from build123d import *

# Parameters (mm, degrees)
BOSS_EXTRUDE1_DEPTH      = 25
CUT_EXTRUDE1_DEPTH       = 4
FILLET1_R                = 4
FILLET2_R                = 10
FILLET3_R                = 5
FILLET4_R                = 3
BOSS_EXTRUDE2_DEPTH      = 3
BOSS_EXTRUDE2_DEPTH_BACK = 3
FILLET5_R                = 3
SKETCH6_W                = 13
SKETCH6_H                = 14
BOSS_EXTRUDE3_DEPTH      = 20
BOSS_EXTRUDE4_DEPTH      = 20
SKETCH9_W                = 13
SKETCH9_H                = 2
BOSS_EXTRUDE5_DEPTH      = 8
SKETCH7_W                = 13
SKETCH7_H                = 2
CUT_EXTRUDE2_DEPTH       = 5
SKETCH11_R               = 1.6
CUT_EXTRUDE3_DEPTH       = 19
CUT_EXTRUDE4_START       = -2
SKETCH12_R               = 1.6
CUT_EXTRUDE4_DEPTH       = 2
CUT_EXTRUDE5_DEPTH       = 6.5
CUT_EXTRUDE5_DEPTH_BACK  = 6.5
CUT_EXTRUDE6_START       = -17
SKETCH15_R               = 6.5
CUT_EXTRUDE6_DEPTH       = 17


with BuildPart() as part:
    # Sketch1 → Boss-Extrude1 (new body)
    with BuildSketch(Plane(origin=(0, 0, 0), x_dir=(0, 0, -1), z_dir=(1, 0, 0))):
        Polygon((0, 0), (-130, 0), (-130, 5), (-100.000366453, 5.148280317), (-77.868517379, 27.5), (101.088229162, 27.5), (114, 18), (114, 0), (74, 0), (74, 7.5), (0, 7.5), align=None)
    extrude(amount=BOSS_EXTRUDE1_DEPTH)

    # Sketch4 → Cut-Extrude1 (cut)
    with BuildSketch(Plane(origin=(25, 0, 0), x_dir=(0, 0, -1), z_dir=(1, 0, 0))):
        Polygon((-100.876178749, 0), (0, 0), (111, 0), (111, 3), (111, 16.482758557), (100.103496394, 24.5), (-76.617181678, 24.5), align=None)
    cut_extrude1 = extrude(amount=-CUT_EXTRUDE1_DEPTH, mode=Mode.SUBTRACT)

    # Mirror2: Cut-Extrude1 across plane
    add(cut_extrude1.mirror(Plane(origin=(12.5, 0, 0), x_dir=(0, 0, 1), z_dir=(1, 0, 0))), mode=Mode.SUBTRACT)

    # Fillet1
    fillet1_edges = [part.edges().sort_by_distance(p)[0] for p in [
        (12.5, 7.5, -74),
        (12.5, 7.5, 0),
    ]]
    fillet(fillet1_edges, radius=FILLET1_R)

    # Fillet2
    fillet2_edges = [part.edges().sort_by_distance(p)[0] for p in [
        (23, 0, 100.876178749),
        (23, 24.5, 76.617181678),
        (23, 24.5, -100.103496394),
        (23, 16.482758557, -111),
        (2, 0, 100.876178749),
        (2, 16.482758557, -111),
        (2, 24.5, -100.103496394),
        (2, 24.5, 76.617181678),
    ]]
    fillet(fillet2_edges, radius=FILLET2_R)

    # Fillet3
    fillet3_edges = [part.edges().sort_by_distance(p)[0] for p in [
        (12.5, 5.148280317, 100.000366453),
        (12.5, 27.5, 77.868517379),
        (12.5, 27.5, -101.088229162),
        (12.5, 18, -114),
    ]]
    fillet(fillet3_edges, radius=FILLET3_R)

    # Fillet4
    fillet4_edges = [part.edges().sort_by_distance(p)[0] for p in [
        (0, 2.5, 130),
        (25, 2.5, 130),
    ]]
    fillet(fillet4_edges, radius=FILLET4_R)

    # Sketch5 → Boss-Extrude2 (add, two sides: drawn at the far end of the back side and taken through both)
    with BuildSketch(Plane(origin=(12.5, 0, 0), x_dir=(0, 0, -1), z_dir=(1, 0, 0)).offset(-BOSS_EXTRUDE2_DEPTH_BACK)):
        Polygon((-117.8659777, 5.059975288), (-103.793914836, 19.271838176), (-72.605250228, 19.271838176), (-95.8659777, 5.059975288), align=None)
    extrude(amount=BOSS_EXTRUDE2_DEPTH + BOSS_EXTRUDE2_DEPTH_BACK)

    # Fillet5
    fillet5_edges = [part.edges().sort_by_distance(p)[0] for p in [
        (12.5, 19.271838176, 103.793914836),
    ]]
    fillet(fillet5_edges, radius=FILLET5_R)

    # Sketch6 → Boss-Extrude3 (add)
    with BuildSketch(Plane.XZ):
        Polygon((0, -111), (4, -111), (4, -93), (21, -93), (21, -111), (25, -111), (25, -114), (0, -114), align=None)
        with Locations((12.5, -102)):
            Rectangle(SKETCH6_W, SKETCH6_H, mode=Mode.SUBTRACT)
    extrude(amount=BOSS_EXTRUDE3_DEPTH)

    # Sketch8 → Boss-Extrude4 (add)
    with BuildSketch(Plane.XZ):
        Polygon((21, 85), (4, 85), (4, 64), (6, 64), (6, 83), (19, 83), (19, 64), (21, 64), align=None)
    extrude(amount=BOSS_EXTRUDE4_DEPTH)

    # Sketch9 → Boss-Extrude5 (add)
    with BuildSketch(Plane.XZ):
        with Locations((12.5, 65)):
            Rectangle(SKETCH9_W, SKETCH9_H)
    extrude(amount=BOSS_EXTRUDE5_DEPTH)

    # Sketch7 → Cut-Extrude2 (cut)
    with BuildSketch(Plane.XZ.offset(20)):
        with Locations((12.5, -94)):
            Rectangle(SKETCH7_W, SKETCH7_H)
    extrude(amount=-CUT_EXTRUDE2_DEPTH, mode=Mode.SUBTRACT)

    # Sketch11 → Cut-Extrude3 (cut)
    with BuildSketch(Plane(origin=(0, 0, -114), x_dir=(-1, 0, 0), z_dir=(0, 0, -1))):
        with Locations((-15.75, -16.25)):
            Circle(SKETCH11_R)
        with Locations((-15.75, -8.75)):
            Circle(SKETCH11_R)
        with Locations((-9.25, -8.75)):
            Circle(SKETCH11_R)
        with Locations((-9.25, -16.25)):
            Circle(SKETCH11_R)
    extrude(amount=-CUT_EXTRUDE3_DEPTH, mode=Mode.SUBTRACT)

    # Sketch12 → Cut-Extrude4 (cut)
    with BuildSketch(Plane.XY.offset(85).offset(CUT_EXTRUDE4_START)):
        with Locations(Location((15.75, -16.25, 0), (0, 0, 180))):
            Circle(SKETCH12_R)
        with Locations(Location((9.25, -16.25, 0), (0, 0, 180))):
            Circle(SKETCH12_R)
        with Locations(Location((9.25, -8.75, 0), (0, 0, 180))):
            Circle(SKETCH12_R)
        with Locations(Location((15.75, -8.75, 0), (0, 0, 180))):
            Circle(SKETCH12_R)
    extrude(amount=CUT_EXTRUDE4_DEPTH, mode=Mode.SUBTRACT)

    # Sketch14 → Cut-Extrude5 (cut, two sides: drawn at the far end of the back side and taken through both)
    with BuildSketch(Plane(origin=(12.5, 0, 0), x_dir=(0, 0, -1), z_dir=(1, 0, 0)).offset(-CUT_EXTRUDE5_DEPTH_BACK)):
        Polygon((-83, 0), (-83, 13.475167258), (-72.975167258, 23.5), (95.592427597, 23.5), (109, 10.092427597), (109, 0), (95, 0), (95, 3.57939317), (87.07939317, 11.5), (-5.825100808, 11.5), (-13.325100808, 4), (-66, 4), (-66, 0), align=None)
    extrude(amount=CUT_EXTRUDE5_DEPTH + CUT_EXTRUDE5_DEPTH_BACK, mode=Mode.SUBTRACT)

    # Sketch15 → Cut-Extrude6 (cut)
    with BuildSketch(Plane.ZY.offset(-4).offset(CUT_EXTRUDE6_START)):
        with Locations((-91, 16)):
            Circle(SKETCH15_R)
        with Locations((-39.333333333, 16)):
            Circle(SKETCH15_R)
        with Locations((64, 16)):
            Circle(SKETCH15_R)
        with Locations((12.333333333, 16)):
            Circle(SKETCH15_R)
    extrude(amount=CUT_EXTRUDE6_DEPTH, mode=Mode.SUBTRACT)


solid = part.part
Build history of the part. All positions in model axes, mm. A direction names the side the tool comes from. Give positions to 0.01 mm unless a question says otherwise; leave off trailing zeros. Order: outer loops, then holes, each group sorted by start corner. A loop starts at its lowest first (then second) coordinate and runs counter-clockwise, first axis right, second up. Notation, with made-up numbers: M 78.25,77.25 L 116.25,77.25 A10 ccw 116.25,95.25 Z; hole C 60.25,84.25 d11. An arc over 180 degrees is marked long. Use one line per item in the form item = value.
1) Probe probe 1 along Z at (x, y) = (13.5, -6); probe 2 along X at (y, z) = (4, 77); probe 3 along Y at (x, z) = (17.5, 34). List the from-to ranges inside material, lowest first.
Calculated:
probe_1 = -114 to -109, -95 to -93, 64 to 66, 83 to 85
probe_2 = 4 to 6, 19 to 21
probe_3 = 0 to 4, 23.5 to 27.5
2) Saw through at A-A (z = 40). Give the cut face in (x, y), plus the area to 3 significant figures.
Calculated:
outline = M 0,24.5 L 4,24.5 L 4,0 L 21,0 L 21,24.5 L 25,24.5 L 25,27.5 L 0,27.5 Z; hole M 6,4 L 19,4 L 19,23.5 L 6,23.5 Z
area = 238 mm2
3) Saw through at C-C (z = -61.5). Give the cut face in (x, y), plus the area to 3 significant figures.
Calculated:
outline = M 0,24.5 L 4,24.5 L 4,7.5 L 21,7.5 L 21,24.5 L 25,24.5 L 25,27.5 L 0,27.5 Z; hole M 6,11.5 L 19,11.5 L 19,23.5 L 6,23.5 Z
area = 208 mm2
4) Two-plate mould, pull along X, no slides. Class faces 6 (the face through (19, 12, -12)), 7 (the face through (9.5, 12, 102)), 8 (the face through (12, 23.5, -10)), 9 (the face through (23, 24.5, -13)): released by +X, released by -X, zero draft, split by the parting line, or undercut.
Calculated:
face_6 = undercut
face_7 = released by -X
face_8 = undercut
face_9 = zero draft
5) Drop flat-ended pins along their axis: pin 1 (10 mm diameter, centred on x = 8, y = -13, fed in from +Z); pin 2 (3 mm diameter, centred on x = 19.5, z = -28.5, fed in from -Y); pin 3 (1.5 mm diameter, centred on x = 10, z = 27, fed in from -Y). Give the stop position or say it passes through.
Calculated:
pin_1 = 85
pin_2 = 7.5
pin_3 = 0
6) Tool access for faces 1 (the face through (12, 0, -84)), 2 (the face through (15.5, 12, 102)), 3 (the face through (13, -10, 85)), 4 (the face through (2.028, 23.708, 76.347)), 5 (the face through (12, 11.5, -15)): list every direction of +Z, -Z, +X, -X, +Y, -Y with a clear straight run to the whole face (end or side of a thin tool).
Calculated:
face_1 = +X, -X, -Y
face_2 = +Z, +X, +Y
face_3 = +Z, +X, -X, -Y
face_4 = -X, -Y
face_5 = none
7) Saw through at B-B (z = -91). Give the cut face in (x, y).
Calculated:
outline = M 0,24.5 L 4,24.5 L 4,22.5 L 6,22.5 L 6,23.5 L 19,23.5 L 19,22.5 L 21,22.5 L 21,24.5 L 25,24.5 L 25,27.5 L 0,27.5 Z; M 4,0 L 21,0 L 21,9.5 L 19,9.5 L 19,7.58 L 6,7.58 L 6,9.5 L 4,9.5 Z
